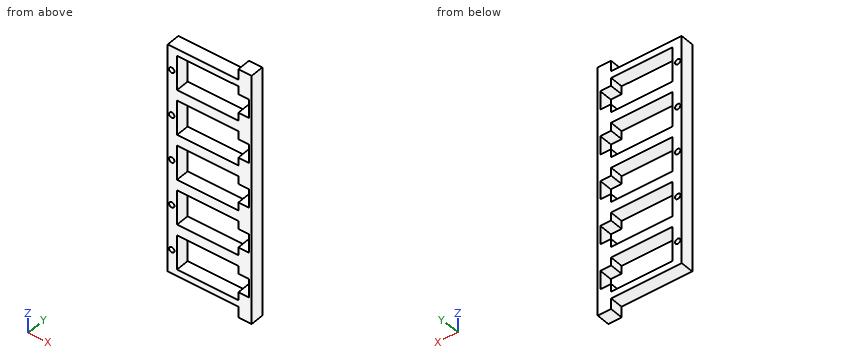
Autodesk Inventor part; units mm, degrees
ref_plane "YZ Plane" through (0, 0, 0) normal (1, 0, 0) x (0, 1, 0)
ref_plane "XZ Plane" through (0, 0, 0) normal (0, 1, 0) x (-1, 0, 0)
ref_plane "XY Plane" through (0, 0, 0) normal (0, 0, 1) x (1, 0, 0)
sketch "Sketch1" plane through (0, 0, 0) normal (0, 1, 0) x (-1, 0, 0)
  line L0 (0, 0) -> (27.5, 0)
  line L1 (27.5, 0) -> (27.5, -2.5)
  line L2 (27.5, -2.5) -> (5, -2.5)
  line L3 (5, -2.5) -> (5, -15.5)
  line L4 (5, -15.5) -> (27.5, -15.5)
  line L5 (27.5, -15.5) -> (27.5, -18)
  line L6 (27.5, -18) -> (0, -18)
  line L7 (0, -18) -> (0, 0)
  line L8 (27.5, -2.5) -> (28, -2.5)
  line L9 (28, -2.5) -> (28, -15.5)
  line L10 (28, -15.5) -> (27.5, -15.5)
  line L11 (27.5, 0) -> (31.5, 0)
  line L12 (31.5, 0) -> (31.5, -18)
  line L13 (31.5, -18) -> (27.5, -18)
  circle A0 centre (30, -9) radius 1
  line L14 (5, -5.5) -> (0, -5.5)
  line L15 (5, -12.5) -> (0, -12.5)
  line L16 (0, 0) -> (0, 4)
  line L17 (0, 4) -> (5, 4)
  line L18 (5, 4) -> (5, 0)
  line L19 (0, -18) -> (0, -22)
  line L20 (0, -22) -> (5, -22)
  line L21 (5, -22) -> (5, -18)
  line L22 (0.9553, -12.5) -> (0.9553, -5.5)
  dimension "d1" = 2.5
  dimension "d2" = 22.5
  dimension "d4" = 2.5
  dimension "d5" = 5
  dimension "d9" = 13
  dimension "d16" = 0.5
  dimension "d17" = 4
  dimension "d19" = 2
  dimension "d20" = 6.5
  dimension "d21" = 3
  dimension "d22" = 3
  dimension "d23" = 4
  dimension "d24" = 4
extrude "Extrusion1" add sketch "Sketch1" along normal blind 5 contours L16 L17 L18 L0 | L0 L1 L2 L3 L14 L7 | L14 L22 L15 L7 | L11 L12 L13 L5 L10 L9 L8 L1 | L15 L3 L4 L5 L6 L7 | L6 L21 L20 L19
pattern_linear "Rectangular Pattern1" count 5 spacing 17 along (0, 0, -1)
properties part number "ServoHolder"
Could you check a few things on this model? Use its own coordinates, in mm. Give positions to 0.01 mm unless a question says otherwise; leave off trailing zeros. Write each loop counter-clockwise with the first axis right and the second up, starting at its lowest first coordinate (ties: lowest second). Pieces come first, ordered by that corner, then holes. Notation, with made-up numbers: (88.5, -18) -> (136.5, -18) arc R13 ccw to (136.5, 6) -> close; hole circle Ø3 at (24, 53.25). An arc over 180 degrees is marked (long way). Answer as a JSON object with one key per item and string values.
Q1. Suppose I cut it at A-A on x = -26.5. Write out the boundary of the cut face in (y, z), then the cut area to 3 significant figures.
Taken from the geometry:
{"outline": "(0, -86) -> (5, -86) -> (5, -83.5) -> (0, -83.5) -> close; (0, -70.5) -> (5, -70.5) -> (5, -66.5) -> (0, -66.5) -> close; (0, -53.5) -> (5, -53.5) -> (5, -49.5) -> (0, -49.5) -> close; (0, -36.5) -> (5, -36.5) -> (5, -32.5) -> (0, -32.5) -> close; (0, -19.5) -> (5, -19.5) -> (5, -15.5) -> (0, -15.5) -> close; (0, -2.5) -> (5, -2.5) -> (5, 0) -> (0, 0) -> close", "area": "105 mm²"}
Q2. Please list where these lines run through material, in increasing order: L1, parallel to Z at x = -7, y = 2.15; L2, parallel to Z at x = -30, y = 2.05; L3, parallel to X at y = 2.95, z = -77.
Taken from the geometry:
{"L1": "z = -86 to -83.5, -70.5 to -66.5, -53.5 to -49.5, -36.5 to -32.5, -19.5 to -15.5, -2.5 to 0", "L2": "z = -86 to -78, -76 to -61, -59 to -44, -42 to -27, -25 to -10, -8 to 0", "L3": "x = -31.5 to -31, -29 to -28, -0.96 to 0"}
Q3. Will this pin go through, and if not, where does the flat tip stop? pin 1 Ø2.5 at (x, y) = (-21, 3.5) entering from +Z.
Taken from the geometry:
{"pin 1": "stops at z = 0"}
Q4. Suppose I cut it at B-B on z = -43. Write out the boundary of the cut face in (x, y), then the cut area to 3 significant figures.
Taken from the geometry:
{"outline": "(-31.5, 0) -> (-31, 0) -> (-31, 5) -> (-31.5, 5) -> close; (-29, 0) -> (-28, 0) -> (-28, 5) -> (-29, 5) -> close; (-0.96, 0) -> (0, 0) -> (0, 5) -> (-0.96, 5) -> close", "area": "12.3 mm²"}
Q5. Suppose I cut it at D-D on y = 2.6. Count the separate pieces of the cut face and the enclosed holes in it, then the cut area to 3 significant figures.
Taken from the geometry:
{"separate pieces": "1", "enclosed holes": "10", "area": "1,100 mm²"}
Q6. Suppose I cut it at C-C on z = -64.5. Write out the boundary of the cut face in (x, y), then the cut area to 3 significant figures.
Taken from the geometry:
{"outline": "(-31.5, 0) -> (-28, 0) -> (-28, 5) -> (-31.5, 5) -> close; (-5, 0) -> (0, 0) -> (0, 5) -> (-5, 5) -> close", "area": "42.5 mm²"}
